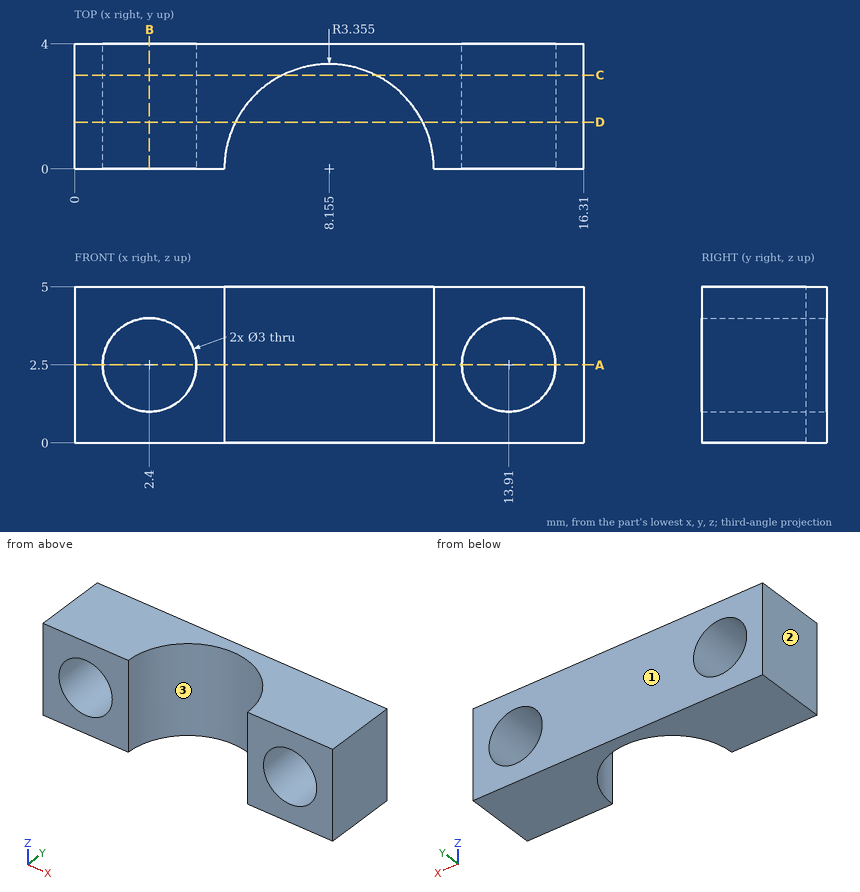
Geometry: see drawing. Coordinates: mm, zero at the bounding-box minimum. Round coordinates to 2 decimals unless told otherwise and drop trailing zeros. Loops run counter-clockwise (first coordinate to the right, second up) from the corner with the lowest first, then second, coordinate; pieces in that order, holes last. Notation, with made-up numbers: (18, 63.25) - (73, 63.25) arc R14 ccw to (73, 70.25) - close; hole circle Ø4 at (-26, 48). An arc over 180 degrees is marked (long way). Use CSV: the item, a comma, the result in double quotes.
Q1. Mould query, pull axis X, two halves, no side actions, for the marked faces 1, 2 and 3. Classes: pulls with the +X half, pulls with the -X half, needs draft (parallel to the pull), parting line crosses it, or undercut.
Reported:
face 1,"needs draft"
face 2,"pulls with the -X half"
face 3,"undercut"
Q2. Section query C-C, the plane y = 3. Output: boundary loops of the cut face in (x, z), then the cut area to 3 significant figures.
Reported:
outline,"(0, 0) - (6.65, 0) - (6.65, 5) - (0, 5) - close; (9.66, 0) - (16.31, 0) - (16.31, 5) - (9.66, 5) - close; hole circle Ø3 at (2.4, 2.5); hole circle Ø3 at (13.91, 2.5)"
area,"52.4 mm^2"
Q3. Section query A-A, the plane z = 2.5. Output: boundary loops of the cut face in (x, y) (3 decimals).
Reported:
outline,"(0, 0) - (0.9, 0) - (0.9, 4) - (0, 4) - close; (3.9, 0) - (4.8, 0) arc R3.355 cw to (11.51, 0) - (12.41, 0) - (12.41, 4) - (3.9, 4) - close; (15.41, 0) - (16.31, 0) - (16.31, 4) - (15.41, 4) - close"
Q4. Ray query, line 1 along Z through (x, y) = (2.4, 1); line 2 along X through (y, z) = (1.75, 2.5); line 3 along X through (y, z) = (1.1, 2.5). Return the intervals inside material, ascending.
Reported:
line 1,"0 to 1, 4 to 5"
line 2,"0 to 0.9, 3.9 to 5.29, 11.02 to 12.41, 15.41 to 16.31"
line 3,"0 to 0.9, 3.9 to 4.99, 11.32 to 12.41, 15.41 to 16.31"
Q5. Section query D-D, the plane y = 1.5. Output: boundary loops of the cut face in (x, z), then the cut area to 3 significant figures.
Reported:
outline,"(0, 0) - (5.15, 0) - (5.15, 5) - (0, 5) - close; (11.16, 0) - (16.31, 0) - (16.31, 5) - (11.16, 5) - close; hole circle Ø3 at (2.4, 2.5); hole circle Ø3 at (13.91, 2.5)"
area,"37.4 mm^2"
Q6. Section query B-B, the plane x = 2.4. Output: boundary loops of the cut face in (y, z), then the cut area to 3 significant figures.
Reported:
outline,"(0, 0) - (4, 0) - (4, 1) - (0, 1) - close; (0, 4) - (4, 4) - (4, 5) - (0, 5) - close"
area,"8.00 mm^2"
